from build123d import *

# Parameters (mm, degrees)
F1_DEPTH       = 5
F2_R           = 21.536165151
F3_DEPTH       = 5.001
F4_W           = 5
F4_H           = 27.6149739623
F5_DEPTH       = 15
F6_R           = 7.62
F7_W           = 5
F7_H           = 7.544119532
F8_DEPTH       = 8.382
F9_R           = 1.5
F10_DEPTH      = 21.078940234
F10_DEPTH_BACK = 28.623059766
F11_W          = 7.3633623496
F11_H          = 12.0904415441
F12_DEPTH      = 6.35
F13_W          = 7.1302087698
F13_H          = 20.9519683909
F14_DEPTH      = 6.35
F15_R          = 6.34999
F16_R          = 5.08


# Not quite as in the source:
# - a fillet or chamfer is up to 0.001 mm smaller than in the source, because OpenCascade refuses the exact size


with BuildPart() as f1:
    # F0 (on Right) → F1 (new body)
    with BuildSketch(Plane.YZ):
        with BuildLine():
            ThreePointArc((0, 6.35), (-4.4901280605, 4.4901280605), (-6.35, 0))
            Line((-6.35, 0), (-6.35, -36.927669698))
            ThreePointArc((-6.35, -36.927669698), (-4.4901280605, -41.4177977585), (0, -43.277669698))
            Line((0, -43.277669698), (37, -43.277669698))
            ThreePointArc((37, -43.277669698), (41.4901280605, -41.4177977585), (43.35, -36.927669698))
            Line((43.35, -36.927669698), (43.35, 0))
            ThreePointArc((43.35, 0), (41.4901280605, 4.4901280605), (37, 6.35))
            Line((37, 6.35), (0, 6.35))
        make_face()
        with BuildLine():
            ThreePointArc((0, -1.5), (-1.0606601718, 1.0606601718), (1.5, 0))
            Line((1.5, 0), (35.5, 0))
            ThreePointArc((35.5, 0), (37, 1.5), (38.5, 0))
            ThreePointArc((38.5, 0), (38.0606601718, -1.0606601718), (37, -1.5))
            Line((37, -1.5), (37, -35.4276701232))
            ThreePointArc((37, -35.4276701232), (38.0606601718, -35.8670099514), (38.5, -36.9276701232))
            ThreePointArc((38.5, -36.9276701232), (37, -38.4276701232), (35.5, -36.9276701232))
            Line((35.5, -36.9276701232), (1.5, -36.9276701232))
            ThreePointArc((1.5, -36.9276701232), (-1.0606601718, -37.988330295), (0, -35.4276701232))
            Line((0, -35.4276701232), (0, -1.5))
        make_face(mode=Mode.SUBTRACT)
        with BuildLine():
            Line((35.5, 0), (1.5, 0))
            ThreePointArc((1.5, 0), (1.0606601718, -1.0606601718), (0, -1.5))
            Line((0, -1.5), (0, -35.4276701232))
            ThreePointArc((0, -35.4276701232), (1.0606601718, -35.8670099514), (1.5, -36.9276701232))
            Line((1.5, -36.9276701232), (35.5, -36.9276701232))
            ThreePointArc((35.5, -36.9276701232), (35.9393398282, -35.8670099514), (37, -35.4276701232))
            Line((37, -35.4276701232), (37, -1.5))
            ThreePointArc((37, -1.5), (35.9393398282, -1.0606601718), (35.5, 0))
        make_face()
    extrude(amount=F1_DEPTH)

    # F2 (on face) → F3 (cut, through all)
    with BuildSketch(Plane.YZ.offset(5)):
        with Locations((19.8611337692, -18.463834849)):
            Circle(F2_R)
    extrude(amount=-F3_DEPTH, mode=Mode.SUBTRACT)

    # F4 (on face) → F5 (join)
    with BuildSketch(Plane.XY.offset(6.35)):
        with Locations((2.5, 18.5)):
            Rectangle(F4_W, F4_H)
    extrude(amount=F5_DEPTH)

    # F6
    f6_edges = [f1.edges().sort_by_distance(p)[0] for p in [
        (2.5, 32.307487, 21.35),
        (2.5, 4.692513, 21.35),
    ]]
    fillet(f6_edges, radius=F6_R)

    # F7 (on face) → F8 (cut)
    with BuildSketch(Plane.XY.offset(21.35)):
        with Locations((2.5, 18.5)):
            Rectangle(F7_W, F7_H)
    extrude(amount=-F8_DEPTH, mode=Mode.SUBTRACT)

    # F9 (on face) → F10 (cut, two sides)
    with BuildSketch(Plane(origin=(0, 14.727940234, 0), x_dir=(-1, 0, 0), z_dir=(0, 1, 0))) as f10_sk:
        with Locations((-2.5, 17.159)):
            Circle(F9_R)
    extrude(amount=-F10_DEPTH, mode=Mode.SUBTRACT)
    extrude(f10_sk.sketch, amount=F10_DEPTH_BACK, mode=Mode.SUBTRACT)

    # F11 (on face) → F12 (cut)
    with BuildSketch(Plane(origin=(0, 32.3074869812, 0), x_dir=(-1, 0, 0), z_dir=(0, 1, 0))):
        with Locations((-1.3183188252, 19.775220772)):
            Rectangle(F11_W, F11_H)
    extrude(amount=-F12_DEPTH, mode=Mode.SUBTRACT)

    # F13 (on face) → F14 (cut)
    with BuildSketch(Plane.XZ.offset(-4.6925130188)):
        with Locations((1.4348956151, 24.2059841955)):
            Rectangle(F13_W, F13_H)
    extrude(amount=-F14_DEPTH, mode=Mode.SUBTRACT)

    # F15 (radius 6.35 in the source; OpenCascade refuses exactly that, so slightly less here)
    f15_edges = [f1.edges().sort_by_distance(p)[0] for p in [
        (2.5, 4.692513, 13.73),
        (2.5, 32.307487, 13.73),
    ]]
    fillet(f15_edges, radius=F15_R)

    # F16
    f16_edges = [f1.edges().sort_by_distance(p)[0] for p in [
        (2.5, 4.692513, 6.35),
        (2.5, 32.307487, 6.35),
    ]]
    fillet(f16_edges, radius=F16_R)


solid = f1.part
Design review of the part built by this model. Coordinates are the model's own, in mm. A direction names the side the tool comes from. Coordinates: 2 decimals unless noted, no trailing zeros. Order: outer loops, then holes, each group sorted by start corner. A loop starts at its lowest first (then second) coordinate and runs counter-clockwise, first axis right, second up. Notation, with made-up numbers: (64, 27.25) -> (110, 27.25) arc R24 cw to (110, 62.25) -> close; hole circle Ø2 at (28.5, 85). An arc over 180 degrees is marked (long way). One line per item, written item: value.
1) We need section B-B, the plane z = -14. Give the boundary of the cut face in (x, y).
Output values:
outline: (0, -6.35) -> (5, -6.35) -> (5, -1.21) -> (0, -1.21) -> close; (0, 40.93) -> (5, 40.93) -> (5, 43.35) -> (0, 43.35) -> close
2) We need section A-A, the plane y = 6.5. Give the boundary of the cut face in (x, z), then the cut area to 3 significant figures.
Output values:
outline: (0, -43.28) -> (5, -43.28) -> (5, -35.35) -> (0, -35.35) -> close; (0, -1.57) -> (5, -1.57) -> (5, 11.82) -> (0, 11.82) -> close
area: 107 mm2
3) Clearance check with flat-ended pins moving along their axes: P1, Ø2.5, axis at x = 2.5, z = 19.5, coming from the -Y side; P2, Ø2, axis at x = 2, y = 4.5, coming from the +Z side; P3, Ø1.5, axis at x = 2, y = 19, coming from the +Z side. State where each tip first meets the part, or that it passes through.
Output values:
P1: stops at y = 11.04
P2: stops at z = 10.48
P3: stops at z = 12.97
4) We need section C-C, the plane x = 3.2. Count the separate pieces of the cut face and the enclosed holes in it, then the cut area to 3 significant figures.
Output values:
separate pieces: 3
enclosed holes: 5
area: 1,170 mm2
5) Draft analysis for pull direction Z (two halves, no side actions). For faces 1 (the face through (2.825, 12.911, 15.695)), 2 (the face through (2.46, -4.44, 4.54)), 3 (the face through (1, 14.728, 18)), state which applies: +Z half, -Z half, draft (parallel to the pull), parting line (faces both ways), or undercut.
Output values:
face 1: undercut
face 2: +Z half
face 3: draft
6) To check wall thickness, follow probe 1 along Y at (x, z) = (2.8, 15); probe 2 along Z at (x, y) = (2.5, 12.8); probe 3 along Z at (x, y) = (4.3, 23). State the ranges of each line that lie inside material, in increasing order. Write a range as [from, to].
Output values:
probe 1: y = [11.04, 14.73], [22.27, 25.96]
probe 2: z = [-43.28, -38.81], [1.88, 15.66], [18.66, 21.35]
probe 3: z = [-43.28, -39.77], [2.84, 21.35]
7) Machinability: for faces 4 (the face through (1, 11.043, 18)), 5 (the face through (2.535, 15.193, -39.488)), 6 (the face through (1, 25.957, 18)), 7 (the face through (2, 19, 12.968)), which of the approach directions +Z, -Z, +X, -X, +Y, -Y give a long, thin tool a straight path to every point of the face, cutting with its end or side? Answer none if there is none.
Output values:
face 4: +Z, +X, -X, -Y
face 5: +X, -X
face 6: +Z, +X, -X, +Y
face 7: +Z, +X, -X
